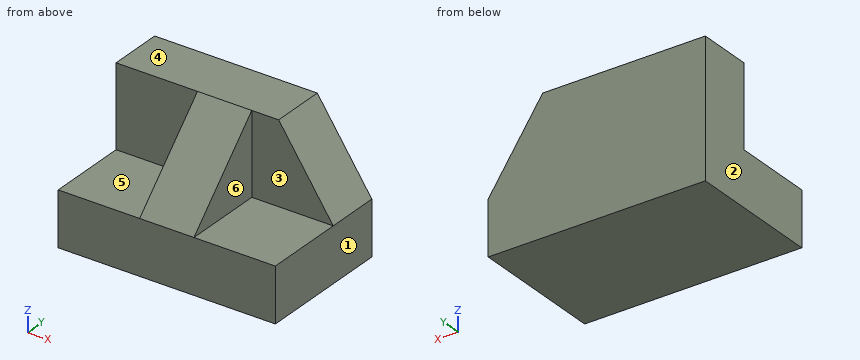
from build123d import *

# Parameters (mm, degrees)
F1_DEPTH = 31.75
F2_W     = 19.05
F2_H     = 19.05
F3_DEPTH = 19.05
F5_DEPTH = 19.05
F7_DEPTH = 25.4


with BuildPart() as f1:
    # F0 (on Front) → F1 (new body)
    with BuildSketch(Plane.XZ):
        Polygon((0, 31.75), (0, 0), (50.8, 0), (50.8, 12.7), (38.039813, 31.75), align=None)
    extrude(amount=F1_DEPTH)

    # F2 (on face) → F3 (cut)
    with BuildSketch(Plane.XZ.offset(31.75)):
        with Locations((9.525, 22.225)):
            Rectangle(F2_W, F2_H)
    extrude(amount=-F3_DEPTH, mode=Mode.SUBTRACT)

    # F4 (on face) → F5 (cut)
    with BuildSketch(Plane.XZ.offset(31.75)):
        Polygon((31.75, 12.7), (50.8, 12.7), (38.039813, 31.75), (31.75, 31.75), align=None)
    extrude(amount=-F5_DEPTH, mode=Mode.SUBTRACT)

    # F6 (on face) → F7 (cut)
    with BuildSketch(Plane.YZ.offset(31.75)):
        Polygon((-31.75, 12.7), (-12.7, 31.75), (-31.75, 31.75), align=None)
    extrude(amount=-F7_DEPTH, mode=Mode.SUBTRACT)


solid = f1.part
Model file for the job. Use its own axes, mm. Face numbers are marked on the shaded views. A direction names the side the tool comes from. Give positions to 0.01 mm unless a question says otherwise; leave off trailing zeros. Order: outer loops, then holes, each group sorted by start corner. A loop starts at its lowest first (then second) coordinate and runs counter-clockwise, first axis right, second up. Notation, with made-up numbers: (75.5, -8) - (119.5, -8) arc R25 cw to (119.5, 31) - close; hole circle Ø10 at (74.25, 89.25). An arc over 180 degrees is marked (long way). Write item = value, one per line. Start each with the question number.
1. Cut at D-D, the plane x = 36. List the corners of the cut face in (y, z).
2. Drop flat-ended pins along their axis: P1, Ø8, axis at y = -23.5, z = 18.5, coming from the -X side; P2, Ø5.5, axis at x = 8.5, y = -18.5, coming from the +Z side; P3, Ø15, axis at x = 6, z = 23.5, coming from the -Y side. Give the stop position or say it passes through.
3. Which spindle directions (+Z, -Z, +X, -X, +Y, -Y) get a long thin tool onto all of the face, cutting with end or side? Do the marked faces 4, 5 and 6. Say none if no direction does.
4. Cut at C-C, the plane z = 22. List the corners of the cut face in (x, y), and give its area (3 significant figures).
5. Two-plate mould, pull along X, no slides. Class the marked faces 1, 2 and 3: pulls with the +X half, pulls with the -X half, needs draft (parallel to the pull), parting line crosses it, or undercut.
6. Cut at B-B, the plane y = -22. List the corners of the cut face in (x, z).
7. Cut at A-A, the plane x = 20.5. List the corners of the cut face in (y, z), and give its area (3 significant figures).
8. Probe line 1 along Z through (x, y) = (39, -17.5); line 2 along Y through (x, z) = (14, 29); line 3 along X through (y, z) = (-17, 20). List the from-to ranges inside material, lowest first.
Taken from the geometry:
q1.outline = (-31.75, 0) - (0, 0) - (0, 31.75) - (-12.7, 31.75) - (-12.7, 12.7) - (-31.75, 12.7) - close
q2.P1 = 19.05
q2.P2 = 12.7
q2.P3 = -12.7
q3.face_4 = +Z, +X, -X, +Y, -Y
q3.face_5 = +Z, -X, -Y
q3.face_6 = +Z, +X, -Y
q4.outline = (0, -12.7) - (19.05, -12.7) - (19.05, -22.45) - (31.75, -22.45) - (31.75, -12.7) - (44.57, -12.7) - (44.57, 0) - (0, 0) - close
q4.area = 690 mm²
q5.face_1 = pulls with the +X half
q5.face_2 = pulls with the -X half
q5.face_3 = needs draft
q6.outline = (0, 0) - (50.8, 0) - (50.8, 12.7) - (31.75, 12.7) - (31.75, 22.45) - (19.05, 22.45) - (19.05, 12.7) - (0, 12.7) - close
q7.outline = (-31.75, 0) - (0, 0) - (0, 31.75) - (-12.7, 31.75) - (-31.75, 12.7) - close
q7.area = 827 mm²
q8.line_1 = 0 to 12.7
q8.line_2 = -12.7 to 0
q8.line_3 = 19.05 to 31.75
